Autodesk Inventor part; units mm, degrees
sketch "草圖1" plane through (0, 0, 0) normal (0, 0, 1) x (1, 0, 0)
  line L0 (0, 0) -> (100, 0)
  line L1 (100, 0) -> (100, 10)
  line L2 (0, 0) -> (0, 10)
  line L3 (0, 10) -> (9, 10)
  line L4 (9, 10) -> (9, 20)
  line L5 (9, 20) -> (15, 20)
  line L6 (15, 20) -> (15, 10)
  line L7 (15, 10) -> (15, 10)
  line L8 (15, 10) -> (15, 5)
  line L9 (15, 5) -> (35, 5)
  line L10 (35, 5) -> (35, 10)
  line L11 (35, 10) -> (45, 10)
  line L12 (45, 10) -> (45, 20)
  line L13 (45, 20) -> (51, 20)
  line L14 (51, 20) -> (51, 10)
  line L15 (51, 10) -> (100, 10)
  dimension "d0" = 100
  dimension "d1" = 10
  dimension "d2" = 10
  dimension "d3" = 9
  dimension "d4" = 10
  dimension "d5" = 6
  dimension "d9" = 5
  dimension "d11" = 20
  dimension "d12" = 10
  dimension "d13" = 6
extrude "擠出1" add sketch "草圖1" along normal blind 50
sketch "草圖2" plane through (9, 20, 0) normal (0, 1, 0) x (1, 0, 0)
  line L0 (0, 0) -> (0, -50)
  line L1 (0, -50) -> (0, -26)
  line L2 (6, -26) -> (6, -24)
  line L3 (0, -26) -> (0, -24)
  line L4 (36, 0) -> (36, -50)
  line L5 (36, -50) -> (36, -26)
  line L6 (36, -26) -> (42, -26)
  line L7 (42, -26) -> (42, -24)
  line L8 (42, -24) -> (36, -24)
  line L9 (36, -26) -> (36, -24)
  line L10 (0, -26) -> (6, -26)
  line L11 (6, -24) -> (0, -24)
  line L12 (0, -26) -> (0, -24)
  point P0 (-9, 0)
  dimension "d16" = 24
  dimension "d17" = 2
  dimension "d18" = 24
  dimension "d19" = 6
  dimension "d22" = 6
  dimension "d27" = 2
extrude "擠出2" cut sketch "草圖2" against normal up to surface (10 mm away) contours L8 L7 L6 L4
extrude "擠出3" cut sketch "草圖2" against normal up to surface (10 mm away) contours L11 L2 L10 L0
sketch "草圖4" plane through (0, 0, 0) normal (0, 1, 0) x (-1, 0, 0)
  line L0 (0, 50) -> (-100, 50)
  line L1 (-100, 50) -> (-100, 38)
  line L2 (-100, 0) -> (-100, 50)
  line L3 (-100, 38) -> (-75.5, 38)
  line L4 (-51, 26) -> (-51, 50)
  line L5 (0, 50) -> (0, 38)
  line L6 (0, 0) -> (0, 50)
  line L7 (0, 38) -> (-4.5, 38)
  dimension "d56" = 12
  dimension "d57" = 24.5
  dimension "d58" = 12
  dimension "d59" = 4.5
hole "孔3" at (75.5, 0, 38) at (4.5, 0, 38) direction (0, 1, 0) diameter 5 end through all
properties part number "wire_setbaseV2"
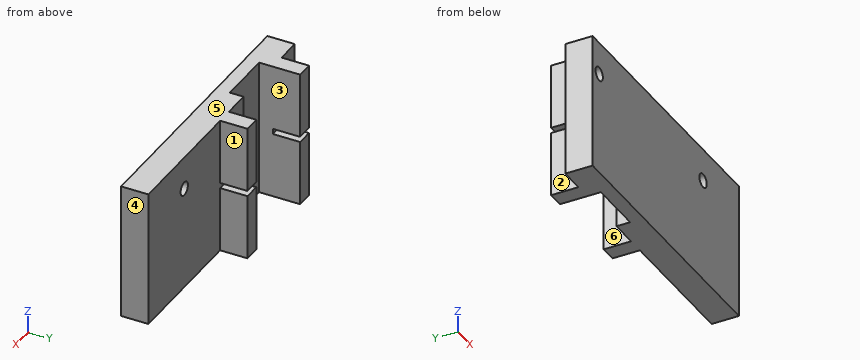
Work out the finished part from the listing and answer in its coordinate system (mm). Face numbers are marked on the shaded views. A direction names the side the tool comes from. Coordinates: 2 decimals unless noted, no trailing zeros. Order: outer loops, then holes, each group sorted by start corner. A loop starts at its lowest first (then second) coordinate and runs counter-clockwise, first axis right, second up. Notation, with made-up numbers: (38, 79.5) - (88, 79.5) arc R28 cw to (88, 107.5) - close; hole circle Ø6 at (-22.75, 82.25). An arc over 180 degrees is marked (long way). Answer as a JSON object with one key per item and string values.
1. A tool of negligible diameter and unlimited length cuts with its end or side. For the marked faces 1, 2 and 3, from which of +Z, -Z, +X, -X, +Y, -Y can it reach the whole face along a straight path? Write none if from no direction.
Output values:
{"face 1": "+Z, -Z, +X, +Y", "face 2": "+Z, -Z, -X, +Y", "face 3": "+Z, -Z, +Y"}
2. Each of these flat-tipped pins is pushed along its axis until it touches: P1, Ø3, axis at y = 13, z = 40.5, coming from the +X side; P2, Ø5, axis at x = 79, y = 8.5, coming from the -Z side; P3, Ø5, axis at y = 15.5, z = 12, coming from the -X side; P4, Ø4.5, axis at x = 4.5, z = 38, coming from the +Y side. Where does it stop, or does it pass through?
Output values:
{"P1": "stops at x = 51", "P2": "stops at z = 0", "P3": "stops at x = 9", "P4": "passes through"}
3. Find section B-B on y = 15. Determine the outline of the cut face in (x, z), plus the area to 3 significant figures.
Output values:
{"outline": "(9, 0) - (15, 0) - (15, 24) - (9, 24) - close; (9, 26) - (15, 26) - (15, 50) - (9, 50) - close; (45, 0) - (51, 0) - (51, 24) - (45, 24) - close; (45, 26) - (51, 26) - (51, 50) - (45, 50) - close", "area": "576 mm²"}
4. The mould has two halves that part along X. Classify the marked faces 4, 5 and 6: +X half, -X half, draft (parallel to the pull), parting line (faces both ways), or undercut.
Output values:
{"face 4": "+X half", "face 5": "draft", "face 6": "undercut"}
5. Consider line 1 (X direction, y = 2, z = 38); line 2 (X direction, y = 7, z = 38); line 3 (Z direction, x = 75.5, y = 6.5). Determine where each line is inside the solid, lowest interval first.
Output values:
{"line 1": "x = 0 to 2, 7 to 73, 78 to 100", "line 2": "x = 0 to 2, 7 to 15, 35 to 73, 78 to 100", "line 3": "z = 0 to 35.5, 40.5 to 50"}
6. Find section D-D on z = 10. Determine the outline of the cut face in (x, y), plus the area to 3 significant figures.
Output values:
{"outline": "(0, 0) - (100, 0) - (100, 10) - (51, 10) - (51, 20) - (45, 20) - (45, 10) - (35, 10) - (35, 5) - (15, 5) - (15, 20) - (9, 20) - (9, 10) - (0, 10) - close", "area": "1,020 mm²"}
7. Find section C-C on x = 75.5. Determine the outline of the cut face in (y, z), plus the area to 3 significant figures.
Output values:
{"outline": "(0, 0) - (10, 0) - (10, 35.5) - (0, 35.5) - close; (0, 40.5) - (10, 40.5) - (10, 50) - (0, 50) - close", "area": "450 mm²"}
8. Find section A-A on z = 38. Determine the outline of the cut face in (x, y).
Output values:
{"outline": "(0, 0) - (2, 0) - (2, 10) - (0, 10) - close; (7, 0) - (73, 0) - (73, 10) - (51, 10) - (51, 20) - (45, 20) - (45, 10) - (35, 10) - (35, 5) - (15, 5) - (15, 20) - (9, 20) - (9, 10) - (7, 10) - close; (78, 0) - (100, 0) - (100, 10) - (78, 10) - close"}
